For this review, take the finished solid that the model builds, in its own axes (mm). A direction names the side the tool comes from. Give positions to 0.01 mm unless a question says otherwise; leave off trailing zeros. Loops run counter-clockwise (first coordinate to the right, second up) from the corner with the lowest first, then second, coordinate; pieces in that order, holes last. Notation, with made-up numbers: (39, 81.5) - (72, 81.5) arc R20 cw to (72, 92.5) - close; hole circle Ø1 at (-17.75, 40). An arc over 180 degrees is marked (long way). Answer as CSV lines item,"result".
from build123d import *

# Parameters (mm, degrees)
PAD_DEPTH    = 0.25
SKETCH001_R  = 0.75
PAD001_DEPTH = 0.25
SKETCH002_R  = 0.75
PAD002_DEPTH = 0.25
SKETCH003_R  = 0.75
PAD003_DEPTH = 0.25
SKETCH004_R  = 0.75
PAD004_DEPTH = 0.4


with BuildPart() as part:
    # Sketch (on DatumPlane) → Pad (new body, symmetric)
    with BuildSketch(Plane.XY.offset(0.5675)):
        Polygon((-7.195606, 5), (-7.195606, 0), (-7.195606, -5), (-6.795606, -5), (-6.395606, -5), (-6.395606, -0.4), (10, -0.4), (10, 0.4), (-6.395606, 0.4), (-6.395606, 5), (-6.795606, 5), align=None)
    extrude(amount=PAD_DEPTH, both=True)

    # Sketch001 (on DatumPlane) → Pad001 (join, symmetric)
    with BuildSketch(Plane.XY.offset(0.5675)):
        Circle(SKETCH001_R)
    extrude(amount=PAD001_DEPTH, both=True)

    # Sketch002 (on DatumPlane) → Pad002 (join, symmetric)
    with BuildSketch(Plane.XY.offset(0.5675)):
        with Locations((-6.795606, 5)):
            Circle(SKETCH002_R)
    extrude(amount=PAD002_DEPTH, both=True)

    # Sketch003 (on DatumPlane) → Pad003 (join, symmetric)
    with BuildSketch(Plane.XY.offset(0.5675)):
        with Locations((-6.795606, -5)):
            Circle(SKETCH003_R)
    extrude(amount=PAD003_DEPTH, both=True)

    # Sphere → Sphere (revolve, cut)
    with BuildSketch(Plane.XZ):
        with BuildLine():
            ThreePointArc((0, -0.635), (0.635, 0), (0, 0.635))
            Line((0, 0.635), (0, -0.635))
        make_face()
    revolve(axis=Axis((0, 0, 0), (0, 0, 1)), mode=Mode.SUBTRACT)

    # Sphere001 → Sphere001 (revolve, cut)
    with BuildSketch(Plane(origin=(-6.795606, 5, 1.135), x_dir=(1, 0, 0), z_dir=(0, -1, 0))):
        with BuildLine():
            ThreePointArc((0, -0.635), (0.635, 0), (0, 0.635))
            Line((0, 0.635), (0, -0.635))
        make_face()
    revolve(axis=Axis((-6.795606, 5, 1.135), (0, 0, 1)), mode=Mode.SUBTRACT)

    # Sphere002 → Sphere002 (revolve, cut)
    with BuildSketch(Plane(origin=(-6.795606, -5, 1.135), x_dir=(1, 0, 0), z_dir=(0, -1, 0))):
        with BuildLine():
            ThreePointArc((0, -0.635), (0.635, 0), (0, 0.635))
            Line((0, 0.635), (0, -0.635))
        make_face()
    revolve(axis=Axis((-6.795606, -5, 1.135), (0, 0, 1)), mode=Mode.SUBTRACT)

    # Sketch004 (on DatumPlane) → Pad004 (join, symmetric)
    with BuildSketch(Plane(origin=(0, 0, 0.5675), x_dir=(1, 0, 0), z_dir=(0, -1, 0))):
        with Locations((6.8, 0)):
            Circle(SKETCH004_R)
    extrude(amount=PAD004_DEPTH, both=True)

    # Sphere003 → Sphere003 (revolve, cut)
    with BuildSketch(Plane(origin=(6.8, 0.7175, 0.5675), x_dir=(1, 0, 0), z_dir=(0, -1, 0))):
        with BuildLine():
            ThreePointArc((0, -0.635), (0.635, 0), (0, 0.635))
            Line((0, 0.635), (0, -0.635))
        make_face()
    revolve(axis=Axis((6.8, 0.7175, 0.5675), (0, 0, 1)), mode=Mode.SUBTRACT)


solid = part.part
1) Draft analysis for pull direction Y (two halves, no side actions). For faces 1 (the flat face through (5.3, -0.4, 0.6)), 2 (the flat face through (5.3, 0.4, 0.6)), 3 (the cylindrical face through (-6.77, 5.75, 0.57)), state which applies: pulls with the +Y half, pulls with the -Y half, needs draft (parallel to the pull), parting line crosses it, or undercut.
From the geometry:
face 1,"pulls with the -Y half"
face 2,"pulls with the +Y half"
face 3,"undercut"
2) Consider section D-D on x = 7. Write out the cut boundary in (y, z).
From the geometry:
outline,"(-0.4, -0.16) - (0.4, -0.16) - (0.4, 0.06) arc R0.6 cw to (0.4, 1.08) - (0.4, 1.29) - (-0.4, 1.29) - close"
3) Wall thickness on line 1 (X direction, y = 1.75, z = 0.5); line 2 (X direction, y = -0.25, z = 0.5); line 3 (X direction, y = 0.5, z = 0.45): over which ranges is each line inside the solid? List them lowest first. Write a range as from..to.
From the geometry:
line 1,"x = -7.2..-6.4"
line 2,"x = -7.2..-0.3, 0.3..10"
line 3,"x = -7.2..-6.4, -0.56..0.56"
4) Consider section C-C on y = 1.5. Write out the cut boundary in (x, z).
From the geometry:
outline,"(-7.2, 0.32) - (-6.4, 0.32) - (-6.4, 0.82) - (-7.2, 0.82) - close"
5) Consider section B-B on x = -5.25. Write out the cut boundary in (y, z), and give its area (3 significant figures).
From the geometry:
outline,"(-0.4, 0.32) - (0.4, 0.32) - (0.4, 0.82) - (-0.4, 0.82) - close"
area,"0.400 mm^2"
6) Insertion check: P1, Ø5, axis at x = 3.5, y = -1.5, coming from the -Z side; P2, Ø0.6, axis at y = 2, z = 0.5, coming from the +X side; P3, Ø3, axis at x = 4, y = 0.5, coming from the +Z side. Each pin has a flat end and moves straight along its axis. Give the tip position at first contact, or say it passes through.
From the geometry:
P1,"stops at z = 0.32"
P2,"stops at x = -6.4"
P3,"stops at z = 0.82"
7) Machinability: for faces 4 (the flat face through (-3, 0, 0.318)), 5 (the cylindrical face through (-6.82, -5.75, 0.57)), 6 (the flat face through (-3, 0, 0.818)), which of the approach directions +Z, -Z, +X, -X, +Y, -Y give a long, thin tool a straight path to every point of the face, cutting with its end or side? Answer none if there is none.
From the geometry:
face 4,"-Z, -X, +Y, -Y"
face 5,"+Z, -Z"
face 6,"+Z, -X, +Y, -Y"
